Autodesk Inventor part; units mm, degrees
ref_plane "YZ Plane" through (0, 0, 0) normal (1, 0, 0) x (0, 1, 0)
ref_plane "XZ Plane" through (0, 0, 0) normal (0, 1, 0) x (-1, 0, 0)
ref_plane "XY Plane" through (0, 0, 0) normal (0, 0, 1) x (1, 0, 0)
sketch "Sketch1" plane through (0, 0, 0) normal (0, 0, 1) x (1, 0, 0)
  line L0 (0, 0) -> (50.8, 0)
  line L1 (50.8, 0) -> (50.8, 76.2)
  line L2 (50.8, 76.2) -> (0, 76.2)
  line L3 (0, 76.2) -> (0, 0)
  line L4 (3.175, 73.025) -> (47.625, 73.025)
  line L5 (47.625, 73.025) -> (47.625, 3.175)
  line L6 (47.625, 3.175) -> (3.175, 3.175)
  line L7 (3.175, 3.175) -> (3.175, 73.025)
  dimension "d13" = 3.175
  dimension "d14" = 50.8
  dimension "d15" = 76.2
  dimension "d37" = 3.175
  dimension "d38" = 3.175
  dimension "d39" = 3.175
extrude "Extrusion1" add sketch "Sketch1" along normal blind 1117.6
hole "Hole1" at (50.8, 38.1, 412.75) direction (-1, 0, 0) diameter 25.4 end through all
hole "Hole2" at (50.8, 38.1, 38.1) direction (-1, 0, 0) diameter 4.7752 end through all
pattern_linear "Rectangular Pattern1" count 3 spacing 158.75 along (0, 0, 1) of "Hole2"
equation "\"d37\" = d13"
equation "\"d38\" = d13"
equation "\"d39\" = d13"
properties part number "GE-12019-02" material "Aluminum-6061"
Could you check a few things on this model? Use its own coordinates, in mm. A direction names the side the tool comes from. Round coordinates to 2 decimals unless told otherwise and drop trailing zeros. Order: outer loops, then holes, each group sorted by start corner. A loop starts at its lowest first (then second) coordinate and runs counter-clockwise, first axis right, second up.
Q1. Thinking about a two-plate mould opening in Z: for faces 1 (the face through (49.19, 34.285, 400.636)), 2 (the face through (3, 41, 1117.6)), 3 (the face through (1.565, 34.285, 400.636)), 4 (the face through (50.8, 38, 551)), which applies, released by +Z, released by -Z, zero draft, split by the parting line, or undercut?
Geometry says:
face 1: undercut
face 2: released by +Z
face 3: undercut
face 4: zero draft
Q2. Imagine slicing it at C-C, the plane z = 646. List the corners of the cut face in (x, y) for me (3 decimals).
Geometry says:
outline: (0, 0) - (50.8, 0) - (50.8, 76.2) - (0, 76.2) - close; hole (3.175, 3.175) - (47.625, 3.175) - (47.625, 73.025) - (3.175, 73.025) - close
Q3. Please list where these lines run through material, in increasing order: probe 1 along Z at (x, y) = (50.1, 38.1); probe 2 along Y at (x, z) = (16, 390.5) (3 decimals); probe 3 along Y at (x, z) = (1, 196).
Geometry says:
probe 1: z = 0 to 35.71, 40.49 to 194.46, 199.24 to 353.21, 357.99 to 400.05, 425.45 to 1117.6
probe 2: y = 0 to 3.175, 73.025 to 76.2
probe 3: y = 0 to 35.87, 40.33 to 76.2
Q4. Which directions (+Z, -Z, +X, -X, +Y, -Y) give clear straight access to the entire face, cutting with the end or side of a thin tool? Please do faces 5 (the face through (47.625, 39, 551)), 6 (the face through (0, 39, 551)).
Geometry says:
face 5: +Z, -Z
face 6: +Z, -Z, -X, +Y, -Y
Q5. Imagine slicing it at B-B, the plane x = 39. List the corners of the cut face in (y, z) for me (3 decimals).
Geometry says:
outline: (0, 0) - (3.175, 0) - (3.175, 1117.6) - (0, 1117.6) - close; (73.025, 0) - (76.2, 0) - (76.2, 1117.6) - (73.025, 1117.6) - close
Q6. Imagine slicing it at A-A, the plane z = 412.75. List the corners of the cut face in (x, y) for me (3 decimals).
Geometry says:
outline: (0, 0) - (50.8, 0) - (50.8, 25.4) - (47.625, 25.4) - (47.625, 3.175) - (3.175, 3.175) - (3.175, 25.4) - (0, 25.4) - close; (0, 50.8) - (3.175, 50.8) - (3.175, 73.025) - (47.625, 73.025) - (47.625, 50.8) - (50.8, 50.8) - (50.8, 76.2) - (0, 76.2) - close
Q7. I'm going to push a flat-ended pin straight in: P1, Ø3, axis at y = 38.1, z = 38.1, coming from the +X side. Where does the tip first touch, or does it pass through?
Geometry says:
P1: passes through
